Can you work these out from the model? Positions are in its coordinate system, mm. A direction names the side the tool comes from. Coordinates: 2 decimals unless noted, no trailing zeros. Order: outer loops, then holes, each group sorted by start corner. A loop starts at its lowest first (then second) coordinate and runs counter-clockwise, first axis right, second up. Notation, with made-up numbers: (-19.75, -5) -> (-7.75, -5) arc R26 cw to (-7.75, 23) -> close; hole circle Ø10 at (63.5, 17). An arc over 180 degrees is marked (long way). Answer in a Markdown table with one row per item.
```python
from build123d import *

# Parameters (mm, degrees)
F0_W      = 79.56
F0_H      = 71.2
F1_DEPTH  = 20
F3_R      = 2
F5_T      = 2
F6_R      = 2
F7_W      = 12.9
F7_H      = 11.5
F8_DEPTH  = 2
F9_W      = 9.9
F9_H      = 11.5
F10_DEPTH = 2
F11_R     = 3.75
F11_R_2   = 1
F12_DEPTH = 4
F13_R     = 1


# Not quite as in the source:
# - a shell that OpenCascade refuses in one call is made with other operations: the cavity is built on its own and cut out


with BuildPart() as f1:
    # F0 (on Top) → F1 (new body)
    with BuildSketch(Plane.XY):
        Rectangle(F0_W, F0_H)
    extrude(amount=F1_DEPTH)

    # F3
    f3_edges = [f1.edges().sort_by_distance(p)[0] for p in [
        (39.78, -35.6, 10),
        (39.78, 35.6, 10),
        (-39.78, 35.6, 10),
        (-39.78, -35.6, 10),
    ]]
    fillet(f3_edges, radius=F3_R)

    # F5: shell of thickness 2, made by hand


with BuildPart() as f5_core1:
    # F5_t2: copy of F1
    add(f1.part)

    # the walls: a layer under each face that stays
    f5_faces = [f5_core1.faces().sort_by_distance(p)[0] for p in [
        (0, 35.6, 10),
        (0, 0, 0),
        (39.78, 0, 10),
        (-39.78, 0, 10),
        (0, -35.6, 10),
    ]]
    thicken(f5_faces, amount=-F5_T, mode=Mode.SUBTRACT)


with BuildPart() as f1_1:
    add(f1.part)

    # what is left inside the walls is the cavity
    f5_cavity = [f5_core1.part.solids().sort_by_distance(p)[0] for p in [
        (0, -11.2, 2.02),
    ]]
    add(f5_cavity, mode=Mode.SUBTRACT)

    # F6
    f6_edges = [f1_1.edges().sort_by_distance(p)[0] for p in [
        (-37.78, 33.6, 11),
        (37.78, 33.6, 11),
        (-37.78, -33.6, 11),
        (37.78, -33.6, 11),
    ]]
    fillet(f6_edges, radius=F6_R)

    # F7 (on face) → F8 (cut)
    with BuildSketch(Plane(origin=(-39.78, 0, 0), x_dir=(0, -1, 0), z_dir=(-1, 0, 0))):
        with Locations((-14.72, 11.25)):
            Rectangle(F7_W, F7_H)
    extrude(amount=-F8_DEPTH, mode=Mode.SUBTRACT)

    # F9 (on face) → F10 (cut)
    with BuildSketch(Plane(origin=(-39.78, 0, 0), x_dir=(0, -1, 0), z_dir=(-1, 0, 0))):
        with Locations((14.08, 11.25)):
            Rectangle(F9_W, F9_H)
    extrude(amount=-F10_DEPTH, mode=Mode.SUBTRACT)

    # F11 (on Top) → F12 (join)
    with BuildSketch(Plane.XY):
        with Locations((-24.28, 24.6)):
            Circle(F11_R)
        with Locations((-24.28, 24.6)):
            Circle(F11_R_2, mode=Mode.SUBTRACT)
        with Locations((27.5, 9.88)):
            Circle(F11_R)
        with Locations((27.5, 9.88)):
            Circle(F11_R_2, mode=Mode.SUBTRACT)
        with Locations((-24.28, -21.6)):
            Circle(F11_R)
        with Locations((-24.28, -21.6)):
            Circle(F11_R_2, mode=Mode.SUBTRACT)
        with Locations((27.5, -16.62)):
            Circle(F11_R)
        with Locations((27.5, -16.62)):
            Circle(F11_R_2, mode=Mode.SUBTRACT)
    extrude(amount=F12_DEPTH)

    # F13
    f13_edges = [f1_1.edges().sort_by_distance(p)[0] for p in [
        (-28.03, 24.6, 2),
        (-28.03, -21.6, 2),
        (23.75, 9.88, 2),
        (23.75, -16.62, 2),
    ]]
    fillet(f13_edges, radius=F13_R)


solid = f1_1.part
```
(1) Suppose I cut it at A-A (y = 9.88). Please give me the cut outline in (x, z).
Response values:
| item | result |
|---|---|
| outline | (-39.78, 0) -> (39.78, 0) -> (39.78, 20) -> (37.78, 20) -> (37.78, 2) -> (32.25, 2) arc R1 cw to (31.25, 3) -> (31.25, 4) -> (28.5, 4) -> (28.5, 2) -> (26.5, 2) -> (26.5, 4) -> (23.75, 4) -> (23.75, 3) arc R1 cw to (22.75, 2) -> (-37.78, 2) -> (-37.78, 5.5) -> (-39.78, 5.5) -> close; (-39.78, 17) -> (-37.78, 17) -> (-37.78, 20) -> (-39.78, 20) -> close |
(2) On a 3-axis mill with a long thin cutter (end or side, diameter ignored), from which of +Z, -Z, +X, -X, +Y, -Y can I reach the whole of each face in a straight line? I mean faces 1 (the flat face through (-39, 15, 5.5)), 2 (the cylindrical face through (39.18, -35.03, 10.14)), 3 (the cylindrical face through (27.3, 8.9, 3)). Say none if no direction works.
Response values:
| item | result |
|---|---|
| face 1 | -X |
| face 2 | +Z, -Z, +X, -Y |
| face 3 | +Z |
(3) Suppose I cut it at B-B (x = 27.5). Please give me the cut outline in (y, z), and give its area (3 significant figures).
Response values:
| item | result |
|---|---|
| outline | (-35.6, 0) -> (35.6, 0) -> (35.6, 20) -> (33.6, 20) -> (33.6, 2) -> (14.63, 2) arc R1 cw to (13.63, 3) -> (13.63, 4) -> (10.88, 4) -> (10.88, 2) -> (8.88, 2) -> (8.88, 4) -> (6.13, 4) -> (6.13, 3) arc R1 cw to (5.13, 2) -> (-11.87, 2) arc R1 cw to (-12.87, 3) -> (-12.87, 4) -> (-15.62, 4) -> (-15.62, 2) -> (-17.62, 2) -> (-17.62, 4) -> (-20.37, 4) -> (-20.37, 3) arc R1 cw to (-21.37, 2) -> (-33.6, 2) -> (-33.6, 20) -> (-35.6, 20) -> close |
| area | 237 mm2 |
(4) I need wall thicknesses on line 1 (Y direction, x = -24.28, z = 3.3); line 2 (Y direction, x = -24.28, z = 2.9); line 3 (X direction, y = -16.62, z = 3.15). Which ranges of each line are inside material? Lowest first, please. Write a range as [from, to].
Response values:
| item | result |
|---|---|
| line 1 | [-35.6, -33.6], [-25.35, -22.6], [-20.6, -17.85], [20.85, 23.6], [25.6, 28.35], [33.6, 35.6] |
| line 2 | [-35.6, -33.6], [-25.36, -22.6], [-20.6, -17.84], [20.84, 23.6], [25.6, 28.36], [33.6, 35.6] |
| line 3 | [-39.78, -37.78], [23.75, 26.5], [28.5, 31.25], [37.78, 39.78] |
(5) Suppose I cut it at D-D (y = -2). Please give me the cut outline in (x, z), and give its area (3 significant figures).
Response values:
| item | result |
|---|---|
| outline | (-39.78, 0) -> (39.78, 0) -> (39.78, 20) -> (37.78, 20) -> (37.78, 2) -> (-37.78, 2) -> (-37.78, 20) -> (-39.78, 20) -> close |
| area | 231 mm2 |
(6) We'd pull the mould along Z, two halves only. Please class faces 4 (the flat face through (-39, 15, 17)), 5 (the flat face through (28.3, -15.7, 4)), 6 (the cylindrical face through (37.18, -33.03, 11.13)): +Z half, -Z half, draft (parallel to the pull), parting line (faces both ways), or undercut.
Response values:
| item | result |
|---|---|
| face 4 | undercut |
| face 5 | +Z half |
| face 6 | draft |
(7) Will these pins go through, and if not, where does the flat tip stop? pin 1 Ø6 at (x, y) = (25.5, 10) entering from +Z; pin 2 Ø8 at (x, y) = (26, 20) entering from +Z; pin 3 Ø1 at (x, z) = (-39.5, 12) entering from -Y.
Response values:
| item | result |
|---|---|
| pin 1 | z = 4 |
| pin 2 | z = 2 |
| pin 3 | y = -35.18 |
(8) Suppose I cut it at C-C (z = 11.5). Please give me the cut outline in (x, y).
Response values:
| item | result |
|---|---|
| outline | (-39.78, -33.6) arc R2 ccw to (-37.78, -35.6) -> (37.78, -35.6) arc R2 ccw to (39.78, -33.6) -> (39.78, 33.6) arc R2 ccw to (37.78, 35.6) -> (-37.78, 35.6) arc R2 ccw to (-39.78, 33.6) -> (-39.78, 21.17) -> (-37.78, 21.17) -> (-37.78, 31.6) arc R2 cw to (-35.78, 33.6) -> (35.78, 33.6) arc R2 cw to (37.78, 31.6) -> (37.78, -31.6) arc R2 cw to (35.78, -33.6) -> (-35.78, -33.6) arc R2 cw to (-37.78, -31.6) -> (-37.78, -19.03) -> (-39.78, -19.03) -> close; (-39.78, -9.13) -> (-37.78, -9.13) -> (-37.78, 8.27) -> (-39.78, 8.27) -> close |
